from build123d import *

# Parameters (mm, degrees)
F0_W     = 59.5203563571
F0_H     = 63.6409893632
F1_DEPTH = 27.2
F3_DEPTH = 29
F5_DEPTH = 23.7


with BuildPart() as f1:
    # F0 (on Top) → F1 (new body, symmetric)
    with BuildSketch(Plane.XY):
        Rectangle(F0_W, F0_H)
    extrude(amount=F1_DEPTH, both=True)

    # F2 (on face) → F3 (join)
    with BuildSketch(Plane(origin=(0, 31.8204946816, 0), x_dir=(-1, 0, 0), z_dir=(0, 1, 0))):
        Polygon((-29.7601781785, -27.2), (-29.7601781785, 27.2), (-52.8728328645, 6.5217590891), (-52.8728328645, -27.2), align=None)
    extrude(amount=-F3_DEPTH)

    # F4 (on face) → F5 (join)
    with BuildSketch(Plane(origin=(-29.7601781785, 0, 0), x_dir=(0, -1, 0), z_dir=(-1, 0, 0))):
        Polygon((31.8204946816, -6.837928202), (31.8204946816, -27.2), (75.0524103642, -27.2), (75.0524103642, -17.8717095405), align=None)
    extrude(amount=-F5_DEPTH)


solid = f1.part
Part model, mm, in its own coordinate system. A direction names the side the tool comes from. Give positions to 0.01 mm unless a question says otherwise; leave off trailing zeros. Loops run counter-clockwise (first coordinate to the right, second up) from the corner with the lowest first, then second, coordinate; pieces in that order, holes last. Notation, with made-up numbers: M -12.75,-12.5 L 22.25,-12.5 A20 cw 22.25,-1.5 Z; hole C -9,-12.5 d8. An arc over 180 degrees is marked long. Put each result on its own line as item: value. Start each with the question number.
1) Saw through at C-C (x = -13). List the corners of the cut face in (y, z).
2) Saw through at B-B (y = 23.5). List the corners of the cut face in (x, z).
3) Saw through at D-D (z = -14). List the corners of the cut face in (x, y).
4) Probe probe 1 along X at (y, z) = (-20, 23); probe 2 along Y at (x, z) = (28, -15.5); probe 3 along Y at (x, z) = (40, 9). List the from-to ranges inside material, lowest first.
5) Flat gauge pins, fed straight in: pin 1 (17.5 mm diameter, centred on y = -7, z = 10, fed in from +X); pin 2 (7 mm diameter, centred on x = 39.5, z = 7, fed in from -Y); pin 3 (10 mm diameter, centred on y = -45, z = -22, fed in from +X). Where does each tip first touch, or does it go through?
6) Saw through at A-A (z = -20). List the corners of the cut face in (x, y), then the cut area to 3 significant figures.
7) 3-axis set-ups, long thin cutter, end or side, ignore diameter. For faces 1 (the flat face through (41.15, 17.52, 17.01)), 2 (the flat face through (0, -31.82, 6)), 3 (the flat face through (-6.06, -48, -19)): which of +Z, -Z, +X, -X, +Y, -Y reach the whole face in a straight line?
Numbers:
1. outline: M -75.05,-27.2 L 31.82,-27.2 L 31.82,27.2 L -31.82,27.2 L -31.82,-6.84 L -75.05,-17.87 Z
2. outline: M -29.76,-27.2 L 52.87,-27.2 L 52.87,6.52 L 29.76,27.2 L -29.76,27.2 Z
3. outline: M -29.76,-59.88 L -6.06,-59.88 L -6.06,-31.82 L 29.76,-31.82 L 29.76,2.82 L 52.87,2.82 L 52.87,31.82 L -29.76,31.82 Z
4. probe 1: -29.76 to 29.76
4. probe 2: -31.82 to 31.82
4. probe 3: 2.82 to 31.82
5. pin 1: x = 29.76
5. pin 2: y = 2.82
5. pin 3: x = -6.06
6. outline: M -29.76,-75.05 L -6.06,-75.05 L -6.06,-31.82 L 29.76,-31.82 L 29.76,2.82 L 52.87,2.82 L 52.87,31.82 L -29.76,31.82 Z
6. area: 5,480 mm^2
7. face 1: +Z, +X, +Y, -Y
7. face 2: +Z, +X, -Y
7. face 3: +Z, -Z, +X, -Y
